Build history of the part. All positions in model axes, mm. A direction names the side the tool comes from. Give positions to 0.01 mm unless a question says otherwise; leave off trailing zeros. Order: outer loops, then holes, each group sorted by start corner. A loop starts at its lowest first (then second) coordinate and runs counter-clockwise, first axis right, second up. Notation, with made-up numbers: (-5, -8.5) - (26, -8.5) arc R22 ccw to (26, 7.5) - close; hole circle Ø2 at (89, 73). An arc over 180 degrees is marked (long way). Answer in a Markdown table with one row per item.
```python
from build123d import *

# Parameters (mm, degrees)
SKETCH1_W           = 4
SKETCH1_H           = 60
BOSS_EXTRUDE1_DEPTH = 50
CUT_EXTRUDE3_REACH  = 81.53
SKETCH2_W           = 17.5
SKETCH2_H           = 25
SKETCH2_W_2         = 3
SKETCH2_H_2         = 17
SKETCH3_R           = 2.75
CUT_EXTRUDE4_DEPTH  = 70.865943062
SKETCH5_W           = 4
SKETCH5_H           = 5
CUT_EXTRUDE5_DEPTH  = 80.529868603
FILLET1_R           = 7


with BuildPart() as part:
    # Sketch1 → Boss-Extrude1 (new body)
    with BuildSketch(Plane.XY):
        with BuildLine():
            Line((4.472135955, 35), (0, 35))
            Line((0, 35), (0, 60))
            Line((0, 60), (-15, 60))
            Line((-15, 60), (-15, 35))
            Line((-15, 35), (-15, -30))
            ThreePointArc((-15, -30), (-13.535533906, -33.535533906), (-10, -35))
            Line((-10, -35), (0, -35))
            ThreePointArc((0, -35), (3.535533906, -33.535533906), (5, -30))
            Line((5, -30), (5, 32.763932023))
            ThreePointArc((5, 32.763932023), (4.866244947, 33.912696625), (4.472135955, 35))
        make_face()
        with Locations((-5.5, 0)):
            Rectangle(SKETCH1_W, SKETCH1_H, mode=Mode.SUBTRACT)
    extrude(amount=BOSS_EXTRUDE1_DEPTH)

    # Sketch2 → Cut-Extrude3 (cut, up to next)
    with BuildSketch(Plane(origin=(0, 0, 0), x_dir=(0, 0, -1), z_dir=(1, 0, 0)), mode=Mode.PRIVATE) as cut_extrude3_sk1:
        with Locations((-8.75, 47.5)):
            Rectangle(SKETCH2_W, SKETCH2_H)
    cut_extrude3_tool1 = extrude(cut_extrude3_sk1.sketch, amount=-CUT_EXTRUDE3_REACH, mode=Mode.PRIVATE) & part.part
    # Sketch2 → Cut-Extrude3 (cut, up to next)
    with BuildSketch(Plane(origin=(0, 0, 0), x_dir=(0, 0, -1), z_dir=(1, 0, 0)), mode=Mode.PRIVATE) as cut_extrude3_sk2:
        with Locations((-41.25, 47.5)):
            Rectangle(SKETCH2_W, SKETCH2_H)
    cut_extrude3_tool2 = extrude(cut_extrude3_sk2.sketch, amount=-CUT_EXTRUDE3_REACH, mode=Mode.PRIVATE) & part.part
    # Sketch2 → Cut-Extrude3 (cut, up to next)
    with BuildSketch(Plane(origin=(0, 0, 0), x_dir=(0, 0, -1), z_dir=(1, 0, 0)), mode=Mode.PRIVATE) as cut_extrude3_sk3:
        with Locations((-28, 51.5)):
            Rectangle(SKETCH2_W_2, SKETCH2_H_2)
    cut_extrude3_tool3 = extrude(cut_extrude3_sk3.sketch, amount=-CUT_EXTRUDE3_REACH, mode=Mode.PRIVATE) & part.part
    # Sketch2 → Cut-Extrude3 (cut, up to next)
    with BuildSketch(Plane(origin=(0, 0, 0), x_dir=(0, 0, -1), z_dir=(1, 0, 0)), mode=Mode.PRIVATE) as cut_extrude3_sk4:
        with Locations((-22, 51.5)):
            Rectangle(SKETCH2_W_2, SKETCH2_H_2)
    cut_extrude3_tool4 = extrude(cut_extrude3_sk4.sketch, amount=-CUT_EXTRUDE3_REACH, mode=Mode.PRIVATE) & part.part
    add(cut_extrude3_tool1.solids().sort_by_distance((0, 47.5, 8.75))[0], mode=Mode.SUBTRACT)
    add(cut_extrude3_tool2.solids().sort_by_distance((0, 47.5, 41.25))[0], mode=Mode.SUBTRACT)
    add(cut_extrude3_tool3.solids().sort_by_distance((0, 51.5, 28))[0], mode=Mode.SUBTRACT)
    add(cut_extrude3_tool4.solids().sort_by_distance((0, 51.5, 22))[0], mode=Mode.SUBTRACT)

    # Sketch3 → Cut-Extrude4 (cut, through all)
    with BuildSketch(Plane.XY.offset(32.5)):
        with Locations((-7.5, 52.5)):
            Circle(SKETCH3_R)
    extrude(amount=-CUT_EXTRUDE4_DEPTH, mode=Mode.SUBTRACT)

    # Sketch5 → Cut-Extrude5 (cut, through all)
    with BuildSketch(Plane.XY.offset(50)):
        with Locations((-5.5, -32.5)):
            Rectangle(SKETCH5_W, SKETCH5_H)
    extrude(amount=-CUT_EXTRUDE5_DEPTH, mode=Mode.SUBTRACT)

    # Fillet1
    fillet1_edges = [part.edges().sort_by_distance(p)[0] for p in [
        (-15, 60, 31),
        (-15, 60, 25),
        (-15, 60, 19),
        (0, 60, 31),
        (0, 60, 25),
        (0, 60, 19),
    ]]
    fillet(fillet1_edges, radius=FILLET1_R)


solid = part.part
```
1. Cut at C-C on y = 54. Write the cut outline in (x, z), and give its area (3 significant figures).
Check result:
| item | result |
|---|---|
| outline | (-14.93, 17.5) - (-9.8, 17.5) - (-9.8, 20.5) - (-14.93, 20.5) - close; (-14.93, 23.5) - (-9.8, 23.5) - (-9.8, 26.5) - (-14.93, 26.5) - close; (-14.93, 29.5) - (-9.8, 29.5) - (-9.8, 32.5) - (-14.93, 32.5) - close; (-5.2, 17.5) - (-0.07, 17.5) - (-0.07, 20.5) - (-5.2, 20.5) - close; (-5.2, 23.5) - (-0.07, 23.5) - (-0.07, 26.5) - (-5.2, 26.5) - close; (-5.2, 29.5) - (-0.07, 29.5) - (-0.07, 32.5) - (-5.2, 32.5) - close |
| area | 92.2 mm² |
2. Cut at A-A on y = -8. Write the cut outline in (x, z).
Check result:
| item | result |
|---|---|
| outline | (-15, 0) - (-7.5, 0) - (-7.5, 50) - (-15, 50) - close; (-3.5, 0) - (5, 0) - (5, 50) - (-3.5, 50) - close |
3. Two-plate mould, pull along X, no slides. Class faces 4 (the face through (-9, -35, 25)), 5 (the face through (-7.5, -3, 25)), 6 (the face through (-2.1, 58, 25)): +X half, -X half, draft (parallel to the pull), parting line (faces both ways), or undercut.
Check result:
| item | result |
|---|---|
| face 4 | draft |
| face 5 | undercut |
| face 6 | +X half |
4. Cut at D-D on x = -11.75. Write the cut outline in (y, z).
Check result:
| item | result |
|---|---|
| outline | (-34.68, 0) - (35, 0) - (35, 17.5) - (58.91, 17.5) - (58.91, 20.5) - (43, 20.5) - (43, 23.5) - (58.91, 23.5) - (58.91, 26.5) - (43, 26.5) - (43, 29.5) - (58.91, 29.5) - (58.91, 32.5) - (35, 32.5) - (35, 50) - (-34.68, 50) - close |
5. Drop flat-ended pins along their axis: P1, Ø12, axis at x = -6.5, y = 47, coming from the -Z side; P2, Ø2.5, axis at x = -10, z = 28, coming from the +Y side; P3, Ø1.5, axis at x = 1.5, z = 38.5, coming from the +Y side; P4, Ø6, axis at x = -8.5, z = 32, coming from the +Y side. Give the stop position or say it passes through.
Check result:
| item | result |
|---|---|
| P1 | stops at z = 17.5 |
| P2 | stops at y = 43 |
| P3 | stops at y = 35 |
| P4 | stops at y = 60 |
6. Probe line 1 (Z direction, x = -2.5, y = 52.5); line 2 (X direction, y = 25, z = 43.5); line 3 (Y direction, x = -7.25, z = 25). List the from-to ranges inside material, lowest first.
Check result:
| item | result |
|---|---|
| line 1 | z = 17.5 to 20.5, 23.5 to 26.5, 29.5 to 32.5 |
| line 2 | x = -15 to -7.5, -3.5 to 5 |
| line 3 | y = 30 to 49.76, 55.24 to 60 |
7. Which spindle directions (+Z, -Z, +X, -X, +Y, -Y) get a long thin tool onto all of the face, cutting with end or side? Do faces 1 (the face through (-6, 30, 25)), 2 (the face through (-7, 47, 32.5)), 3 (the face through (-7, 43, 22)). Say none if no direction does.
Check result:
| item | result |
|---|---|
| face 1 | +Z, -Z, -Y |
| face 2 | +Z, +X, -X, +Y |
| face 3 | +X, -X, +Y |
8. Cut at B-B on z = 4.5. Write the cut outline in (x, y), and give its area (3 significant figures).
Check result:
| item | result |
|---|---|
| outline | (-15, -30) arc R5 ccw to (-10, -35) - (-7.5, -35) - (-7.5, 30) - (-3.5, 30) - (-3.5, -35) - (0, -35) arc R5 ccw to (5, -30) - (5, 32.76) arc R5 ccw to (4.47, 35) - (-15, 35) - close |
| area | 1,130 mm² |
